Can you work these out from the model? Positions are in its coordinate system, mm. Give positions to 0.01 mm unless a question says otherwise; leave off trailing zeros. Loops run counter-clockwise (first coordinate to the right, second up) from the corner with the lowest first, then second, coordinate; pieces in that order, holes last. Notation, with made-up numbers: (85.25, 10.25) - (102.25, 10.25) arc R18 cw to (102.25, 19.25) - close; hole circle Ø4 at (74.5, -5). An arc over 180 degrees is marked (long way). Answer in a Markdown table with one row per item.
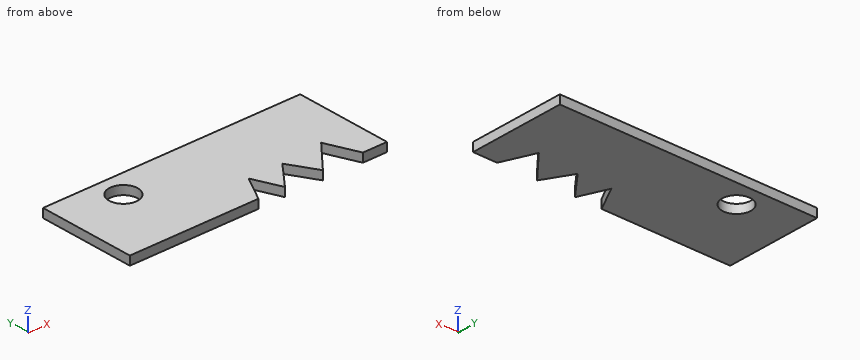
from build123d import *

# Parameters (mm, degrees)
F0_W     = 88.67468
F0_H     = 33.368226
F1_DEPTH = 3
F2_R     = 4.914899
F3_DEPTH = 25
F5_DEPTH = 25


with BuildPart() as f1:
    # F0 (on Top) → F1 (new body)
    with BuildSketch(Plane.XY):
        Rectangle(F0_W, F0_H)
    extrude(amount=F1_DEPTH)

    # F2 (on face) → F3 (cut)
    with BuildSketch(Plane.XY.offset(3)):
        with Locations((-24.283957, 8.138201)):
            Circle(F2_R)
    extrude(amount=-F3_DEPTH, mode=Mode.SUBTRACT)

    # F4 (on face) → F5 (cut)
    with BuildSketch(Plane.XY.offset(3)):
        Polygon((5.171371, -7.167339), (0, -16.684113), (18.780243, -47.993954), (36.018144, -16.684113), (31.481858, -5.715726), (22.227822, -16.684113), (16.784273, -7.167339), (9.163308, -16.684113), align=None)
    extrude(amount=-F5_DEPTH, mode=Mode.SUBTRACT)


solid = f1.part
Q1. Imagine slicing it at D-D, the plane x = 35. Write out the boundary of the cut face in (y, z).
Checked values:
| item | result |
|---|---|
| outline | (-14.22, 0) - (16.68, 0) - (16.68, 3) - (-14.22, 3) - close |
Q2. Imagine slicing it at B-B, the plane y = 11.5. Write out the boundary of the cut face in (x, z), and give its area (3 significant figures).
Checked values:
| item | result |
|---|---|
| outline | (-44.34, 0) - (-27.87, 0) - (-27.87, 3) - (-44.34, 3) - close; (-20.7, 0) - (44.34, 0) - (44.34, 3) - (-20.7, 3) - close |
| area | 245 mm² |
Q3. Imagine slicing it at C-C, the plane z = 2.1. Write out the boundary of the cut face in (x, y).
Checked values:
| item | result |
|---|---|
| outline | (-44.34, -16.68) - (0, -16.68) - (5.17, -7.17) - (9.16, -16.68) - (16.78, -7.17) - (22.23, -16.68) - (31.48, -5.72) - (36.02, -16.68) - (44.34, -16.68) - (44.34, 16.68) - (-44.34, 16.68) - close; hole circle Ø9.83 at (-24.28, 8.14) |
Q4. Imagine slicing it at A-A, the plane y = -12.5. Write out the boundary of the cut face in (x, z), and give its area (3 significant figures).
Checked values:
| item | result |
|---|---|
| outline | (-44.34, 0) - (2.27, 0) - (2.27, 3) - (-44.34, 3) - close; (7.41, 0) - (12.51, 0) - (12.51, 3) - (7.41, 3) - close; (19.83, 0) - (25.76, 0) - (25.76, 3) - (19.83, 3) - close; (34.29, 0) - (44.34, 0) - (44.34, 3) - (34.29, 3) - close |
| area | 203 mm² |
Q5. For pin 1 (8 mm diameter, centred on x = -22, y = 4.5, fed in from -Z), with a flat end and sliding along its axis, tell me the tip position at first contact or that it passes through.
Checked values:
| item | result |
|---|---|
| pin 1 | stops at z = 0 |
Q6. If I drill on line 1 (X direction, y = -10.5, z = 2.45); line 2 (X direction, y = -11, z = 1.85); line 3 (X direction, y = 5, z = 0.4), over which ranges is the centre line in solid material (lowest first)? Write a range as [from, to].
Checked values:
| item | result |
|---|---|
| line 1 | x = [-44.34, 3.36], [6.57, 14.12], [18.69, 27.45], [33.46, 44.34] |
| line 2 | x = [-44.34, 3.09], [6.78, 13.72], [18.98, 27.02], [33.67, 44.34] |
| line 3 | x = [-44.34, -28.07], [-20.5, 44.34] |
